```python
from build123d import *

# Parameters (mm, degrees)
ESQUISSE1_R        = 1.5
BOSS_EXTRU_1_DEPTH = 5


with BuildPart() as part:
    # Esquisse1 → Boss.-Extru.1 (new body)
    with BuildSketch(Plane.XY):
        with BuildLine():
            Line((0, 0), (26.277186767, 0))
            ThreePointArc((26.277186767, 0), (55, 15), (83.722813233, 0))
            Line((83.722813233, 0), (90, 0))
            Line((90, 0), (90, 31))
            Line((90, 31), (85, 31))
            Line((85, 31), (85, 41))
            Line((85, 41), (90, 41))
            Line((90, 41), (90, 46))
            Line((90, 46), (85, 46))
            Line((85, 46), (85, 56))
            Line((85, 56), (90, 56))
            Line((90, 56), (90, 61))
            Line((90, 61), (0, 61))
            Line((0, 61), (0, 56))
            Line((0, 56), (5, 56))
            Line((5, 56), (5, 46))
            Line((5, 46), (0, 46))
            Line((0, 46), (0, 41))
            Line((0, 41), (5, 41))
            Line((5, 41), (5, 31))
            Line((5, 31), (0, 31))
            Line((0, 31), (0, 0))
        make_face()
        with Locations((85, 20)):
            Circle(ESQUISSE1_R, mode=Mode.SUBTRACT)
        with Locations((15, 20)):
            Circle(ESQUISSE1_R, mode=Mode.SUBTRACT)
    extrude(amount=BOSS_EXTRU_1_DEPTH)


solid = part.part
```
Geometry: final body of the model. Coordinates: model frame, mm. A direction names the side the tool comes from. Give positions to 0.01 mm unless a question says otherwise; leave off trailing zeros. Write each loop counter-clockwise with the first axis right and the second up, starting at its lowest first coordinate (ties: lowest second). Pieces come first, ordered by that corner, then holes.
1. Section query C-C, the plane x = 15. Return loops of the section in (y, z), then the cut area to 3 significant figures.
2. Section query B-B, the plane z = 4. Return loops of the section in (x, y), then the cut area to 3 significant figures.
3. Draft query along Y for faces 4 (the flat face through (87, 0, 2)), 5 (the flat face through (88, 46, 2)), 6 (the flat face through (0, 59, 2)), 7 (the flat face through (88, 31, 2)). Return one class per face: released by +Y, released by -Y, zero draft, split by the parting line, or undercut.
4. Section query D-D, the plane y = 4. Return loops of the section in (x, z), then the cut area to 3 significant figures.
5. Section query A-A, the plane y = 20. Return loops of the section in (x, z), then the cut area to 3 significant figures.
6. Reachability of faces 1 (the flat face through (87, 56, 2)), 2 (the flat face through (44, 31, 0)), 3 (the flat face through (3, 46, 2)) from +Z, -Z, +X, -X, +Y, -Y: full face, straight path, thin tool, end or side. Return the list, or none.
7. Line query: probe 1 along Y at (x, z) = (15, 2.45); probe 2 along X at (y, z) = (40.5, 4.6); probe 3 along Y at (x, z) = (30.5, 2.85) (3 decimals). Output: solid intervals per line, ascending.
8. Pin query (flat end, axial travel): P1, Ø2.5, axis at y = 53, z = 1.5, coming from the -X side; P2, Ø1.5, axis at y = 51, z = 3.5, coming from the +X side. Return the tip coordinate at first contact, or that it passes through.
Computed:
1. outline: (0, 0) - (18.5, 0) - (18.5, 5) - (0, 5) - close; (21.5, 0) - (61, 0) - (61, 5) - (21.5, 5) - close
1. area: 290 mm2
2. outline: (0, 0) - (26.28, 0) arc R35 cw to (83.72, 0) - (90, 0) - (90, 31) - (85, 31) - (85, 41) - (90, 41) - (90, 46) - (85, 46) - (85, 56) - (90, 56) - (90, 61) - (0, 61) - (0, 56) - (5, 56) - (5, 46) - (0, 46) - (0, 41) - (5, 41) - (5, 31) - (0, 31) - close; hole circle Ø3 at (15, 20); hole circle Ø3 at (85, 20)
2. area: 4,670 mm2
3. face 4: released by -Y
3. face 5: undercut
3. face 6: zero draft
3. face 7: undercut
4. outline: (0, 0) - (29.52, 0) - (29.52, 5) - (0, 5) - close; (80.48, 0) - (90, 0) - (90, 5) - (80.48, 5) - close
4. area: 195 mm2
5. outline: (0, 0) - (13.5, 0) - (13.5, 5) - (0, 5) - close; (16.5, 0) - (83.5, 0) - (83.5, 5) - (16.5, 5) - close; (86.5, 0) - (90, 0) - (90, 5) - (86.5, 5) - close
5. area: 420 mm2
6. face 1: +Z, -Z, +X
6. face 2: -Z, +X, -X, +Y, -Y
6. face 3: +Z, -Z, -X
7. probe 1: y = 0 to 18.5, 21.5 to 61
7. probe 2: x = 5 to 85
7. probe 3: y = 4.995 to 61
8. P1: stops at x = 5
8. P2: stops at x = 85
